```python
from build123d import *

# Parameters (mm, degrees)
EXTRUDE_1_DEPTH = 20
SKETCH_2_W      = 16
SKETCH_2_H      = 8
SKETCH_2_R      = 2.502951076
EXTRUDE_2_DEPTH = 3
EXTRUDE_START   = -3
SKETCH_3_W      = 36
SKETCH_3_H      = 3
EXTRUDE_3_DEPTH = 58
CHAMFER_1_SIZE  = 1


with BuildPart() as part:
    # 草图1 → 凸台-拉伸1 (new body)
    with BuildSketch(Plane(origin=(0, 0, 0), x_dir=(1, 0, 0), z_dir=(0, 1, 0))):
        Polygon((-3, 3), (18.5, 3), (18.5, -3), (15.5, -3), (15.5, 0), (0, 0), (0, -3), (-3, -3), align=None)
    extrude(amount=EXTRUDE_1_DEPTH)

    # 草图2 → 凸台-拉伸2 (add)
    with BuildSketch(Plane.XY.offset(3)):
        with Locations((-11, 8)):
            Rectangle(SKETCH_2_W, SKETCH_2_H)
        with Locations((-14.001123559, 8.002728821)):
            Circle(SKETCH_2_R, mode=Mode.SUBTRACT)
    extrude(amount=-EXTRUDE_2_DEPTH)

    # 草图3 → 凸台-拉伸3 (add)
    with BuildSketch(Plane(origin=(0, 0, -3), x_dir=(-1, 0, 0), z_dir=(0, 0, -1)).offset(EXTRUDE_START)):
        with Locations((-12, 21.5)):
            Rectangle(SKETCH_3_W, SKETCH_3_H)
    extrude(amount=EXTRUDE_3_DEPTH)

    # 倒角1
    chamfer_1_edges = [part.edges().sort_by_distance(p)[0] for p in [
        (30, 23, -29),
        (30, 21.5, -58),
        (30, 20, -29),
        (30, 21.5, 0),
        (-6, 20, -29),
        (-6, 21.5, -58),
        (-6, 23, -29),
        (-6, 21.5, 0),
        (-16.504074634, 8.002728821, 3),
        (-3, 4, 1.5),
        (-3, 12, 1.5),
        (-19, 12, 1.5),
        (-19, 4, 1.5),
        (-19, 8, 0),
        (-11, 4, 0),
        (-11, 12, 0),
        (-3, 8, 0),
        (-3, 20, -1.5),
        (18.5, 20, -1.5),
        (7.75, 0, 0),
        (15.5, 0, 1.5),
        (17, 0, 3),
        (18.5, 0, 0),
        (7.75, 0, -3),
        (0, 0, 1.5),
        (-1.5, 0, 3),
        (-3, 0, 0),
        (-3, 10, -3),
        (18.5, 10, -3),
        (7.75, 20, -3),
    ]]
    chamfer(chamfer_1_edges, length=CHAMFER_1_SIZE)


solid = part.part
```
Build history of the part. All positions in model axes, mm. A direction names the side the tool comes from. Coordinates: 2 decimals unless noted, no trailing zeros. Write each loop counter-clockwise with the first axis right and the second up, starting at its lowest first coordinate (ties: lowest second). Pieces come first, ordered by that corner, then holes.
1. Band-saw the part on B-B, the plane x = 14.5. Give the cut face in (y, z).
Answer block:
outline: (0, -2) - (1, -3) - (19, -3) - (20, -4) - (20, -58) - (23, -58) - (23, 0) - (1, 0) - (0, -1) - close
2. Band-saw the part on C-C, the plane z = -13.5. Give the cut face in (x, y).
Answer block:
outline: (-6, 21) - (-5, 20) - (29, 20) - (30, 21) - (30, 22) - (29, 23) - (-5, 23) - (-6, 22) - close
3. Pull direction Y, two halves, no side cores. Call faces 1 (the cylindrical face through (-11.69, 7.04, 1.01)), 2 (the flat face through (12, 20, -29)), 3 (the flat face through (-3.4, 11.8, 0.2)), 4 (the flat face through (15.5, 10, 2)): released by +Y, released by -Y, zero draft, split by the parting line, or undercut.
Answer block:
face 1: undercut
face 2: released by -Y
face 3: undercut
face 4: zero draft
4. Band-saw the part on A-A, the plane y = 17. Give the cut face in (x, z), and give its area (3 significant figures).
Answer block:
outline: (-3, -2) - (-2, -3) - (17.5, -3) - (18.5, -2) - (18.5, 3) - (15.5, 3) - (15.5, 0) - (0, 0) - (0, 3) - (-3, 3) - close
area: 81.5 mm2
5. 3-axis set-ups, long thin cutter, end or side, ignore diameter. For faces 5 (the flat face through (0, 10, 1)), 6 (the flat face through (8, 10, -3)), 7 (the flat face through (17, 20, 1)), 8 (the flat face through (-11, 4, 2)): which of +Z, -Z, +X, -X, +Y, -Y reach the whole face in a straight line?
Answer block:
face 5: +Z, +Y, -Y
face 6: -Z, +X, -X, -Y
face 7: +Z, +X, -X, +Y
face 8: +Z, -Z, -X, -Y
6. Band-saw the part on D-D, the plane x = 24. Give the cut face in (y, z).
Answer block:
outline: (20, -58) - (23, -58) - (23, 0) - (20, 0) - close
7. Drop flat-ended pins along their axis: pin 1 (17 mm diameter, centred on x = 4.5, z = -29.5, fed in from -Y); pin 2 (5 mm diameter, centred on x = -13.5, y = 7, fed in from -Z); pin 3 (1 mm diameter, centred on x = 10, y = 14.5, fed in from +Z). Give the stop position or say it passes through.
Answer block:
pin 1: stops at y = 20
pin 2: stops at z = 0
pin 3: stops at z = 0
8. Drill centre lines: probe 1 along Y at (x, z) = (23, -15.5); probe 2 along X at (y, z) = (21.25, -41.5); probe 3 along Z at (x, y) = (16, 21.5). Where is each one in solid material? Low to high.
Answer block:
probe 1: y = 20 to 23
probe 2: x = -6 to 30
probe 3: z = -58 to 0
